Model file for the job. Use its own axes, mm. A direction names the side the tool comes from. Round coordinates to 2 decimals unless told otherwise and drop trailing zeros. Loops run counter-clockwise (first coordinate to the right, second up) from the corner with the lowest first, then second, coordinate; pieces in that order, holes last. Notation, with made-up numbers: (-14, 6) - (37, 6) arc R13 ccw to (37, 22) - close; hole circle Ø11 at (39, 68.25). An arc over 180 degrees is marked (long way). Use one line per item in the form item = value.
from build123d import *

# Parameters (mm, degrees)
F0_W     = 29.6
F0_H     = 5
F0_H_2   = 10
F1_DEPTH = 4
F3_DEPTH = 29.6
F4_R     = 3
F5_DEPTH = 33
F6_W     = 29.6
F6_H     = 4
F7_DEPTH = 3
F8_R     = 2
F9_DEPTH = 25


with BuildPart() as f1:
    # F0 (on Top) → F1 (new body)
    with BuildSketch(Plane.XY):
        with Locations((0, 7.5)):
            Rectangle(F0_W, F0_H)
        Rectangle(F0_W, F0_H_2)
        with Locations((0, -7.5)):
            Rectangle(F0_W, F0_H)
    extrude(amount=F1_DEPTH)

    # F2 (on face) → F3 (join)
    with BuildSketch(Plane(origin=(-14.8, 0, 0), x_dir=(0, -1, 0), z_dir=(-1, 0, 0))):
        with BuildLine():
            Line((-6.011283, 4), (10, 4))
            ThreePointArc((10, 4), (1.994358, 12.005642), (-6.011283, 4))
        make_face()
    extrude(amount=-F3_DEPTH)

    # F4 (on face) → F5 (cut)
    with BuildSketch(Plane(origin=(-14.8, 0, 0), x_dir=(0, -1, 0), z_dir=(-1, 0, 0))):
        with Locations((2, 6)):
            Circle(F4_R)
    extrude(amount=-F5_DEPTH, mode=Mode.SUBTRACT)

    # F6 (on face) → F7 (join)
    with BuildSketch(Plane(origin=(0, 10, 0), x_dir=(-1, 0, 0), z_dir=(0, 1, 0))):
        with Locations((0, 2)):
            Rectangle(F6_W, F6_H)
    extrude(amount=F7_DEPTH)

    # F8 (on face) → F9 (cut)
    with BuildSketch(Plane.XY.offset(4)):
        with Locations((0, 9.511283)):
            Circle(F8_R)
    extrude(amount=-F9_DEPTH, mode=Mode.SUBTRACT)


solid = f1.part
1. Tool access for faces 1 (the flat face through (0, 7, 4)), 2 (the flat face through (14.8, 1, 5)): list every direction of +Z, -Z, +X, -X, +Y, -Y with a clear straight run to the whole face (end or side of a thin tool).
Geometry check:
face_1 = +Z, +X, -X, +Y
face_2 = +Z, -Z, +X, +Y, -Y
2. Cut at B-B, the plane y = -2. Give the cut face in (x, z), plus the area to 3 significant figures.
Geometry check:
outline = (-14.8, 0) - (14.8, 0) - (14.8, 3) - (-14.8, 3) - close; (-14.8, 9) - (14.8, 9) - (14.8, 12.01) - (-14.8, 12.01) - close
area = 178 mm^2
3. Wall check: probe 1 along Z at (x, y) = (-0.25, -2); probe 2 along Y at (x, z) = (0, 2.3); probe 3 along Z at (x, y) = (-7, -4.75). Give the ranges that are in metal, low to high.
Geometry check:
probe_1 = 0 to 3, 9 to 12.01
probe_2 = -10 to 7.51, 11.51 to 13
probe_3 = 0 to 4.8, 7.2 to 11.52
4. Cut at C-C, the plane z = 1.5. Give the cut face in (x, y).
Geometry check:
outline = (-14.8, -10) - (14.8, -10) - (14.8, 13) - (-14.8, 13) - close; hole circle Ø4 at (0, 9.51)
5. Pull direction Y, two halves, no side cores. Call faces 3 (the cylindrical face through (-0.207, -2.17, 12.004)), 4 (the cylindrical face through (-0.26, 11.494, 2.028)), 5 (the flat face through (0, 1, 0)): +Y half, -Y half, draft (parallel to the pull), parting line (faces both ways), or undercut.
Geometry check:
face_3 = parting line
face_4 = undercut
face_5 = draft
6. Flat gauge pins, fed straight in: pin 1 (5.5 mm diameter, centred on x = -5.5, y = 10.5, fed in from +Z); pin 2 (2 mm diameter, centred on x = 2.5, y = -4, fed in from +Z); pin 3 (6 mm diameter, centred on x = -8.5, z = 9.5, fed in from -Y). Where does each tip first touch, or does it go through?
Geometry check:
pin_1 = 4
pin_2 = 11.94
pin_3 = -9.6
7. Cut at D-D, the plane z = 6. Give the cut face in (x, y), plus the area to 3 significant figures.
Geometry check:
outline = (-14.8, -9.75) - (14.8, -9.75) - (14.8, -5) - (-14.8, -5) - close; (-14.8, 1) - (14.8, 1) - (14.8, 5.76) - (-14.8, 5.76) - close
area = 281 mm^2
